Read the model definition and answer for the solid it produces. Units are mm, in the model's axes. A direction names the side the tool comes from. Coordinates: 2 decimals unless noted, no trailing zeros. Write each loop counter-clockwise with the first axis right and the second up, starting at its lowest first coordinate (ties: lowest second). Pieces come first, ordered by that corner, then holes. Notation, with made-up numbers: (54, 16.5) -> (98, 16.5) arc R36 ccw to (98, 52.5) -> close; hole circle Ø10 at (-9.5, 4). An arc over 180 degrees is marked (long way). Answer in a Markdown table with one row per item. Add a question column.
Item 1: Section C-C on z = -136.5 is taken. Write down the section's boundary in (x, y).
Item 2: Straight lines are drawn through the part: line 1 (Z direction, x = -169.5, y = 19.5); line 2 (X direction, y = 13.5, z = -231.5); line 3 (X direction, y = 12, z = -178). For each, find the intervals that lie inside material, in ascending order. Write a range as from..to.
Item 3: Which of the six approach directions +Z, -Z, +X, -X, +Y, -Y give full straight-line access (tool end or side, diameter ignored) to faces 5 (the face through (-228.98, 14.93, -133.39)), 6 (the face through (-179.538, 17.535, -199.075))?
Item 4: Section D-D on x = -152.5 is taken. Write down the section's boundary in (y, z).
Item 5: Section A-A on y = 17 is taken. Count the separate pieces of the cut face and the enclosed holes in it, then the cut area to 3 significant figures.
Item 6: For a pull along X with two mould halves and no side action, classify faces 1 (the face through (-242.226, 15.07, -127.199)), 2 (the face through (-128.97, 14.93, -247.41)), 3 (the face through (-124.385, 15.07, -244.182)), 4 (the face through (-189, 20, -189)) as +X half, -X half, draft (parallel to the pull), parting line (faces both ways), or undercut.
Item 7: Section B-B on x = -129.5 is taken. Write down the section's boundary in (y, z), then the cut area to 3 significant figures.
Item 8: Given pin 1 Ø4 at (x, y) = (-155.5, 18) entering from +Z; pin 2 Ø5 at (x, z) = (-222, -140) entering from +Y; pin 3 Ø3 at (y, z) = (14.5, -160) entering from +X; pin 4 Ø2.5 at (x, z) = (-182, -195.5) entering from +Y, each flat-ended and moving along its own axis, determine where each tip first touches the part or whether it passes through.
```python
from build123d import *

# Parameters (mm, degrees)
SKETCH_1_R               = 275
SKETCH_1_R_2             = 255
EXTRUDE_1_DEPTH          = 10
EXTRUDE_2_DEPTH          = 10
SKETCH_8_R               = 2.65
SKETCH_8_R_2             = 1.65
SKETCH_8_R_3             = 2.15
CUT_EXTRUDE_1_DEPTH      = 21
SKETCH_9_OUTSIDE_W       = 707.614
SKETCH_9_OUTSIDE_H       = 707.614
CUT_EXTRUDE_2_DEPTH      = 21
SKETCH_10_W              = 777.504065726
SKETCH_10_H              = 20
CUT_EXTRUDE_3_DEPTH      = 276
CUT_EXTRUDE_3_DEPTH_BACK = 276
EXTRUDE_3_DEPTH          = 10
CUT_EXTRUDE_4_DEPTH      = 10
SKETCH_13_R              = 1.65
CUT_EXTRUDE_5_DEPTH      = 10
CUT_EXTRUDE_START        = -10
SKETCH_14_R              = 4
CUT_EXTRUDE_6_DEPTH      = 5
FILLET_1_R               = 5


with BuildPart() as part:
    # 草图1 → 凸台-拉伸1 (new body)
    with BuildSketch(Plane(origin=(0, 0, 0), x_dir=(1, 0, 0), z_dir=(0, 1, 0))):
        Circle(SKETCH_1_R)
        Circle(SKETCH_1_R_2, mode=Mode.SUBTRACT)
    extrude(amount=EXTRUDE_1_DEPTH)

    # 草图10 → 切除-拉伸3 (cut, two sides)
    with BuildSketch(Plane.XY) as cut_extrude_3_sk:
        Rectangle(SKETCH_10_W, SKETCH_10_H)
    extrude(amount=CUT_EXTRUDE_3_DEPTH, mode=Mode.SUBTRACT)
    extrude(cut_extrude_3_sk.sketch, amount=-CUT_EXTRUDE_3_DEPTH_BACK, mode=Mode.SUBTRACT)


with BuildPart() as body_2:
    # 草图2 → 凸台-拉伸2 (new body)
    with BuildSketch(Plane(origin=(0, 10, 0), x_dir=(1, 0, 0), z_dir=(0, 1, 0))):
        with BuildLine():
            Line((-110.525139894, 257.262887824), (-25.423255477, 200))
            Line((-25.423255477, 200), (0, 200))
            Line((0, 200), (25.423255477, 200))
            Line((25.423255477, 200), (110.525139894, 257.262887824))
            ThreePointArc((110.525139894, 257.262887824), (197.989898732, 197.989898732), (257.262887824, 110.525139894))
            Line((257.262887824, 110.525139894), (200, 25.423255477))
            Line((200, 25.423255477), (200, 0))
            Line((200, 0), (200, -25.423255477))
            Line((200, -25.423255477), (257.262887824, -110.525139894))
            ThreePointArc((257.262887824, -110.525139894), (197.989898732, -197.989898732), (110.525139894, -257.262887824))
            Line((110.525139894, -257.262887824), (25.423255477, -200))
            Line((25.423255477, -200), (0, -200))
            Line((0, -200), (-25.423255477, -200))
            Line((-25.423255477, -200), (-110.525139894, -257.262887824))
            ThreePointArc((-110.525139894, -257.262887824), (-197.989898732, -197.989898732), (-257.262887824, -110.525139894))
            Line((-257.262887824, -110.525139894), (-200, -25.423255477))
            Line((-200, -25.423255477), (-200, 25.423255477))
            Line((-200, 25.423255477), (-257.262887824, 110.525139894))
            ThreePointArc((-257.262887824, 110.525139894), (-197.989898732, 197.989898732), (-110.525139894, 257.262887824))
        make_face()
        with BuildLine():
            Line((0, 185), (30, 185))
            Line((30, 185), (111.993839361, 240.171563565))
            ThreePointArc((111.993839361, 240.171563565), (187.383297014, 187.383297014), (240.171563565, 111.993839361))
            Line((240.171563565, 111.993839361), (185, 30))
            Line((185, 30), (185, 0))
            Line((185, 0), (185, -30))
            Line((185, -30), (240.171563565, -111.993839361))
            ThreePointArc((240.171563565, -111.993839361), (187.383297014, -187.383297014), (111.993839361, -240.171563565))
            Line((111.993839361, -240.171563565), (30, -185))
            Line((30, -185), (0, -185))
            Line((0, -185), (-30, -185))
            Line((-30, -185), (-111.993839361, -240.171563565))
            ThreePointArc((-111.993839361, -240.171563565), (-187.383297014, -187.383297014), (-240.171563565, -111.993839361))
            Line((-240.171563565, -111.993839361), (-185, -30))
            Line((-185, -30), (-185, 30))
            Line((-185, 30), (-240.171563565, 111.993839361))
            ThreePointArc((-240.171563565, 111.993839361), (-187.383297014, 187.383297014), (-111.993839361, 240.171563565))
            Line((-111.993839361, 240.171563565), (-30, 185))
            Line((-30, 185), (0, 185))
        make_face(mode=Mode.SUBTRACT)
    extrude(amount=EXTRUDE_2_DEPTH)

    # 草图8 → 切除-拉伸1 (cut, through all)
    with BuildSketch(Plane(origin=(0, 20, 0), x_dir=(1, 0, 0), z_dir=(0, 1, 0))):
        with Locations((-10, 192.5)):
            Circle(SKETCH_8_R)
        with Locations((10, 192.5)):
            Circle(SKETCH_8_R)
        with Locations((-10, -192.5)):
            Circle(SKETCH_8_R)
        with Locations((10, -192.5)):
            Circle(SKETCH_8_R)
        with Locations((192.5, 10)):
            Circle(SKETCH_8_R)
        with Locations((192.5, -10)):
            Circle(SKETCH_8_R)
        with Locations((-192.5, 10)):
            Circle(SKETCH_8_R)
        with Locations((-192.5, -10)):
            Circle(SKETCH_8_R)
        with Locations((-110.525139894, 248.223100485)):
            Circle(SKETCH_8_R_2)
        with Locations((-27.711627738, 192.5)):
            Circle(SKETCH_8_R_3)
        with Locations((-44.304938442, 203.665215623)):
            Circle(SKETCH_8_R_3)
        with Locations((-56.749921469, 212.03912734)):
            Circle(SKETCH_8_R_3)
        with Locations((-69.194904497, 220.413039057)):
            Circle(SKETCH_8_R_3)
        with Locations((-81.639887524, 228.786950774)):
            Circle(SKETCH_8_R_3)
        with Locations((-146.077022117, 230.028561882)):
            Circle(SKETCH_8_R)
        with Locations((-164.415519771, 217.299729706)):
            Circle(SKETCH_8_R)
        with Locations((-183.638937552, 201.316607082)):
            Circle(SKETCH_8_R)
        with Locations((-201.316607082, 183.638937552)):
            Circle(SKETCH_8_R)
        with Locations((-217.299729706, 164.415519771)):
            Circle(SKETCH_8_R)
        with Locations((-230.028561882, 146.077022117)):
            Circle(SKETCH_8_R)
        with Locations((-128.811575358, 240.123330241)):
            Circle(SKETCH_8_R)
        with Locations((-240.123330241, 128.811575358)):
            Circle(SKETCH_8_R)
        with Locations((-228.786950774, 81.639887524)):
            Circle(SKETCH_8_R_3)
        with Locations((-220.413039057, 69.194904497)):
            Circle(SKETCH_8_R_3)
        with Locations((-212.03912734, 56.749921469)):
            Circle(SKETCH_8_R_3)
        with Locations((-203.665215623, 44.304938442)):
            Circle(SKETCH_8_R_3)
        with Locations((-192.5, 27.711627738)):
            Circle(SKETCH_8_R_3)
        with Locations((-248.223100485, 110.525139894)):
            Circle(SKETCH_8_R_2)
        with Locations((192.5, 27.711627738)):
            Circle(SKETCH_8_R_3)
        with Locations((248.223100485, 110.525139894)):
            Circle(SKETCH_8_R_2)
        with Locations((203.665215623, 44.304938442)):
            Circle(SKETCH_8_R_3)
        with Locations((212.03912734, 56.749921469)):
            Circle(SKETCH_8_R_3)
        with Locations((220.413039057, 69.194904497)):
            Circle(SKETCH_8_R_3)
        with Locations((228.786950774, 81.639887524)):
            Circle(SKETCH_8_R_3)
        with Locations((240.123330241, 128.811575358)):
            Circle(SKETCH_8_R)
        with Locations((230.028561882, 146.077022117)):
            Circle(SKETCH_8_R)
        with Locations((128.811575358, 240.123330241)):
            Circle(SKETCH_8_R)
        with Locations((201.316607082, 183.638937552)):
            Circle(SKETCH_8_R)
        with Locations((183.638937552, 201.316607082)):
            Circle(SKETCH_8_R)
        with Locations((164.415519771, 217.299729706)):
            Circle(SKETCH_8_R)
        with Locations((146.077022117, 230.028561882)):
            Circle(SKETCH_8_R)
        with Locations((81.639887524, 228.786950774)):
            Circle(SKETCH_8_R_3)
        with Locations((69.194904497, 220.413039057)):
            Circle(SKETCH_8_R_3)
        with Locations((56.749921469, 212.03912734)):
            Circle(SKETCH_8_R_3)
        with Locations((44.304938442, 203.665215623)):
            Circle(SKETCH_8_R_3)
        with Locations((110.525139894, 248.223100485)):
            Circle(SKETCH_8_R_2)
        with Locations((27.711627738, 192.5)):
            Circle(SKETCH_8_R_3)
        with Locations((217.299729706, 164.415519771)):
            Circle(SKETCH_8_R)
    extrude(amount=-CUT_EXTRUDE_1_DEPTH, mode=Mode.SUBTRACT)

    # 草图9 outside → 切除-拉伸2 (cut, through all)
    with BuildSketch(Plane(origin=(0, 20, 0), x_dir=(1, 0, 0), z_dir=(0, 1, 0))):
        Rectangle(SKETCH_9_OUTSIDE_W, SKETCH_9_OUTSIDE_H)
        with BuildLine():
            Line((-128.813345638, 248.610381894), (-117.653354647, 237.450390904))
            ThreePointArc((-117.653354647, 237.450390904), (-187.383297014, 187.383297014), (-237.450390904, 117.653354647))
            Line((-237.450390904, 117.653354647), (-248.610381894, 128.813345638))
            ThreePointArc((-248.610381894, 128.813345638), (-197.989898732, 197.989898732), (-128.813345638, 248.610381894))
        make_face(mode=Mode.SUBTRACT)
    extrude(amount=-CUT_EXTRUDE_2_DEPTH, mode=Mode.SUBTRACT)

    # 草图11 → 凸台-拉伸3 (add)
    with BuildSketch(Plane(origin=(0, 20, 0), x_dir=(1, 0, 0), z_dir=(0, 1, 0))):
        Polygon((-222.749556316, 143.553596823), (-233.587670194, 154.391710701), (-154.391710701, 233.587670194), (-143.553596823, 222.749556316), align=None)
    extrude(amount=-EXTRUDE_3_DEPTH)

    # 草图12 → 切除-拉伸4 (cut)
    with BuildSketch(Plane(origin=(0, 20, 0), x_dir=(1, 0, 0), z_dir=(0, 1, 0))):
        with BuildLine():
            Line((-233.587670194, 154.391710701), (-154.391710701, 233.587670194))
            ThreePointArc((-154.391710701, 233.587670194), (-197.989898732, 197.989898732), (-233.587670194, 154.391710701))
        make_face()
    extrude(amount=-CUT_EXTRUDE_4_DEPTH, mode=Mode.SUBTRACT)

    # 草图13 → 切除-拉伸5 (cut)
    with BuildSketch(Plane(origin=(0, 20, 0), x_dir=(1, 0, 0), z_dir=(0, 1, 0))):
        with Locations((-195.525945241, 181.383809617)):
            Circle(SKETCH_13_R)
        with Locations((-206.132546958, 170.777207899)):
            Circle(SKETCH_13_R)
        with Locations((-216.739148676, 160.170606181)):
            Circle(SKETCH_13_R)
        with Locations((-181.383809617, 195.525945241)):
            Circle(SKETCH_13_R)
        with Locations((-170.777207899, 206.132546958)):
            Circle(SKETCH_13_R)
        with Locations((-160.170606181, 216.739148676)):
            Circle(SKETCH_13_R)
    extrude(amount=-CUT_EXTRUDE_5_DEPTH, mode=Mode.SUBTRACT)

    # 草图14 → 切除-拉伸6 (cut)
    with BuildSketch(Plane.XZ.offset(-10).offset(CUT_EXTRUDE_START)):
        with Locations((-181.383809617, -195.525945241)):
            Circle(SKETCH_14_R)
        with Locations((-195.525945241, -181.383809617)):
            Circle(SKETCH_14_R)
    extrude(amount=CUT_EXTRUDE_6_DEPTH, mode=Mode.SUBTRACT)

    # 圆角1
    fillet_1_edges = [body_2.edges().sort_by_distance(p)[0] for p in [
        (-237.450390904, 15, -117.653354647),
        (-117.653354647, 15, -237.450390904),
        (-128.813345638, 15, -248.610381894),
        (-248.610381894, 15, -128.813345638),
        (-143.553596823, 15, -222.749556316),
        (-222.749556316, 15, -143.553596823),
        (-154.391710701, 15, -233.587670194),
        (-233.587670194, 15, -154.391710701),
    ]]
    fillet(fillet_1_edges, radius=FILLET_1_R)


solid = body_2.part
```
Results below:
| question | item | result |
|---|---|---|
| 1 | outline | (-244.47, 10) -> (-227.14, 10) -> (-227.14, 20) -> (-244.47, 20) -> close |
| 2 | line 1 | z = -218.48..-207.18, -205.09..-196.8 |
| 2 | line 2 | x = -156.48..-148.28, -143.87..-128.97 |
| 2 | line 3 | x = -209.98..-188.3 |
| 3 | face 5 | +Z, +X, +Y, -Y |
| 3 | face 6 | +Y |
| 4 | outline | (10, -234.83) -> (20, -234.83) -> (20, -213.8) -> (10, -213.8) -> close |
| 5 | separate pieces | 1 |
| 5 | enclosed holes | 10 |
| 5 | area | 2,360 mm2 |
| 6 | face 1 | undercut |
| 6 | face 2 | parting line |
| 6 | face 3 | +X half |
| 6 | face 4 | draft |
| 7 | outline | (10, -247.46) -> (20, -247.46) -> (20, -242.68) -> (10, -242.68) -> close; (10, -237.56) -> (20, -237.56) -> (20, -231.2) -> (10, -231.2) -> close |
| 7 | area | 111 mm2 |
| 8 | pin 1 | stops at z = -208.8 |
| 8 | pin 2 | passes through |
| 8 | pin 3 | stops at x = -204.8 |
| 8 | pin 4 | stops at y = 15 |
